The listing builds one solid part. Answer for the finished solid, in the listing's coordinates (mm). A direction names the side the tool comes from. Give positions to 0.01 mm unless a question says otherwise; leave off trailing zeros. Write each loop counter-clockwise with the first axis right and the second up, starting at its lowest first coordinate (ties: lowest second). Pieces come first, ordered by that corner, then holes. Notation, with made-up numbers: (78, 79.5) -> (87, 79.5) arc R12 cw to (87, 101.5) -> close; hole circle Ø7 at (66.25, 89). An arc over 180 degrees is marked (long way). Put each result on its own line as item: value. Start each with the question number.
1) A cutting plane is placed at B-B (z = -14). Write down the section's boundary in (x, y), then the cut area to 3 significant figures.
2) A cutting plane is placed at A-A (x = 7.5). Write down the section's boundary in (y, z), then the cut area to 3 significant figures.
3) Find the intervals of material crossed by line 1 along X through (y, z) = (-17, 2); line 2 along X through (y, z) = (-12, -4); line 3 along Z through (x, y) = (19.25, -25.5), in increasing order. Write a range as from..to.
4) For faces 4 (the flat face through (3, -14, -10)), 5 (the flat face through (0, -12, -8)), determine the directions among +Z, -Z, +X, -X, +Y, -Y from which every point of the face is accessible in a straight line to the end or side of a thin tool.
5) A cutting plane is placed at D-D (x = 16.25). Write down the section's boundary in (y, z), then the cut area to 3 significant figures.
6) A flat-ended cylindrical pin translates along its axis: pin 1 Ø3 at (x, y) = (9.5, -17.5) entering from -Z. Find the tip coordinate at first contact, or state that the pin passes through.
7) For a pull along X with two mould halves and no side action, classify faces 1 (the flat face through (15, 0, -11)), 2 (the flat face through (30, -11, -8)), 3 (the cylindrical face through (20.765, -17.228, 2.644)) as released by +X, released by -X, zero draft, split by the parting line, or undercut.
8) A cutting plane is placed at C-C (y = -20.5). Write down the section's boundary in (x, z).
Autodesk Inventor part; units mm, degrees
ref_plane "YZ Plane" through (0, 0, 0) normal (1, 0, 0) x (0, 1, 0)
ref_plane "XZ Plane" through (0, 0, 0) normal (0, 1, 0) x (-1, 0, 0)
ref_plane "XY Plane" through (0, 0, 0) normal (0, 0, 1) x (1, 0, 0)
sketch "Boceto1" plane through (0, 0, 0) normal (0, 0, 1) x (1, 0, 0)
  line L0 (0, 0) -> (30, 0)
  line L1 (30, 0) -> (30, -30)
  line L2 (30, -30) -> (0, -30)
  line L3 (0, -30) -> (0, 0)
  dimension "d0" = 30
  dimension "d1" = 30
extrude "Extrusión1" add sketch "Boceto1" along normal blind 4
sketch "Boceto2" plane through (0, 0, 0) normal (0, 1, 0) x (1, 0, 0)
  line L0 (30, -4) -> (0, -4)
  line L1 (0, -4) -> (30, -4)
  line L2 (30, -4) -> (30, 26)
  line L3 (30, 26) -> (0, 26)
  line L4 (0, 26) -> (0, -4)
  point P0 (0, 0)
  dimension "d4" = 30
extrude "Extrusión2" add sketch "Boceto2" against normal blind 4
sketch "Boceto3" plane through (0, 0, 0) normal (0, 0, -1) x (-1, 0, 0)
  line L0 (0, -4) -> (-30, -4)
  line L1 (-30, -30) -> (-30, -4)
  line L2 (0, -30) -> (-30, -30)
  line L3 (0, -4) -> (0, -30)
  line L4 (0, -30) -> (-30, -30)
  line L5 (-15, -30) -> (-15, -4)
  line L6 (0, -4) -> (0, -30)
  line L7 (0, -17) -> (-30, -17)
  line L8 (-30, -17) -> (-22.5, -17)
  circle A0 centre (-22.5, -17) radius 3
  line L9 (0, -17) -> (-7.5, -17)
  circle A1 centre (-7.5, -17) radius 3
  point P0 (0, 0)
  dimension "d7" = 7.5
  dimension "d8" = 6
  dimension "d9" = 7.5
  dimension "d10" = 6
hole "Agujero1" at (22.5, -17, 0) at (7.5, -17, 0) direction (0, 0, 1) diameter 3.5 end through all countersink diameter 6 countersink angle 90
sketch "Boceto4" plane through (0, 0, 0) normal (0, 0, -1) x (-1, 0, 0)
  line L0 (0, -30) -> (-30, -30)
  line L1 (0, 0) -> (-3, 0)
  line L2 (-3, 0) -> (-3, -30)
  line L3 (-3, -30) -> (0, -30)
  line L4 (0, -30) -> (0, 0)
  line L5 (-30, -30) -> (-27, -30)
  line L6 (-27, -30) -> (-27, 0)
  line L7 (-27, 0) -> (-30, 0)
  line L8 (-30, 0) -> (-30, -30)
  dimension "d18" = 3
  dimension "d19" = 3
extrude "Extrusión3" add sketch "Boceto4" along normal up to surface (26 mm away)
sketch "Boceto5" plane through (30, -30, 4) normal (1, 0, 0) x (0, 0, -1)
  line L0 (30, 26) -> (4, 0)
  line L1 (30, 30) -> (0, 30)
  line L2 (0, 0) -> (0, 30)
  line L3 (30, 0) -> (0, 0)
  line L4 (30, 30) -> (30, 0)
  point P0 (4, 30)
extrude "Extrusión4" cut sketch "Boceto5" against normal through all contours L4 L3 L0
properties part number "Union"
Reply:
1. outline: (0, -16) -> (3, -16) -> (3, -4) -> (27, -4) -> (27, -16) -> (30, -16) -> (30, 0) -> (0, 0) -> close
1. area: 192 mm2
2. outline: (-30, 0) -> (-20, 0) -> (-18.75, 1.25) -> (-18.75, 4) -> (-30, 4) -> close; (-15.25, 1.25) -> (-14, 0) -> (-4, 0) -> (-4, -26) -> (0, -26) -> (0, 4) -> (-15.25, 4) -> close
2. area: 208 mm2
3. line 1: x = 0..5.75, 9.25..20.75, 24.25..30
3. line 2: x = 0..3, 27..30
3. line 3: z = 0..4
4. face 4: -Z, -Y
4. face 5: +Z, -Z, -X, +Y, -Y
5. outline: (-30, 0) -> (-4, 0) -> (-4, -26) -> (0, -26) -> (0, 4) -> (-30, 4) -> close
5. area: 224 mm2
6. pin 1: stops at z = 0
7. face 1: zero draft
7. face 2: released by +X
7. face 3: undercut
8. outline: (0, -9.5) -> (3, -9.5) -> (3, 0) -> (27, 0) -> (27, -9.5) -> (30, -9.5) -> (30, 4) -> (0, 4) -> close
